Can you work these out from the model? Positions are in its coordinate system, mm. A direction names the side the tool comes from. Coordinates: 2 decimals unless noted, no trailing zeros. Loops run counter-clockwise (first coordinate to the right, second up) from the corner with the lowest first, then second, coordinate; pieces in that order, holes last. Notation, with made-up numbers: (83, 19.5) -> (133, 19.5) arc R5 ccw to (133, 23.5) -> close; hole circle Ø11 at (28.25, 18). An arc over 180 degrees is marked (long way). Put each result on its own line as item: value. Start each with the question number.
Item 1: Please list where these lines run through material, in increasing order: L1, parallel to X at y = 0, z = 13.75 (3 decimals); L2, parallel to X at y = -10, z = 15 (3 decimals); L3, parallel to Y at x = 48, z = 1.25 (3 decimals). Write a range as from..to.
Item 2: If we section it at D-D on x = -11.5: Please give me the cut outline in (y, z) (3 decimals).
Item 3: We'd pull the mould along Y, two halves only. Please class faces 6 (the flat face through (2.85, -26.07, 9.39)), 7 (the flat face through (-55.245, 1, 9)), 8 (the flat face through (1, 41.275, 9)), 9 (the flat face through (9.8, -46.06, 9.39)): pulls with the +Y half, pulls with the -Y half, needs draft (parallel to the pull), parting line crosses it, or undercut.
Item 4: Will these pins go through, and if not, where does the flat tip stop? P1, Ø4, axis at x = 46, z = 11.5, coming from the -Y side (3 decimals); P2, Ø8, axis at y = 17.5, z = 12, coming from the +X side.
Item 5: If we section it at A-A on x = -44.5: Please give me the cut outline in (y, z) (3 decimals), plus the area to 3 significant figures.
Item 6: If we section it at B-B on y = 25: Please give me the cut outline in (x, z) (3 decimals), plus the area to 3 significant figures.
Item 7: For faces 1 (the flat face through (35, -41.275, 9)), 2 (the flat face through (-39, -41.275, 9)), 3 (the flat face through (11.83, -25.95, 9.39)), 4 (the flat face through (20, 3, 0)), 5 (the flat face through (20, 3, 19.05)), which set-ups out of +Z, -Z, +X, -X, +Y, -Y let a thin tool reach every point of the face, with its end or its side?
Item 8: If we section it at C-C on z = 10.5: Please give me the cut outline in (x, y) (3 decimals).
```python
from build123d import *

# Parameters (mm, degrees)
F1_DEPTH = 19.05


with BuildPart() as f1:
    # F0 (on Top) → F1 (new body)
    with BuildSketch(Plane.XY):
        with BuildLine():
            ThreePointArc((95.083343, 10.795), (80.32549, 32.78101), (55.245, 41.275))
            Line((55.245, 41.275), (-55.245, 41.275))
            Line((-55.245, 41.275), (-55.245, -41.275))
            Line((-55.245, -41.275), (-21.336, -41.275))
            Line((-21.336, -41.275), (-7.865616, -41.275))
            Line((-7.865616, -41.275), (-20.82424, -28.316376))
            ThreePointArc((-20.82424, -28.316376), (-23.518744, 28.236761), (-17.489888, -28.058625))
            Line((-17.489888, -28.058625), (-4.273513, -41.275))
            Line((-4.273513, -41.275), (5.155756, -50.704269))
            Line((5.155756, -50.704269), (14.585024, -41.275))
            Line((14.585024, -41.275), (55.245, -41.275))
            ThreePointArc((55.245, -41.275), (80.32549, -32.78101), (95.083343, -10.795))
            ThreePointArc((95.083343, -10.795), (96.52, 0), (95.083343, 10.795))
        make_face()
        Polygon((16.381076, -30.498693), (7.40082, -39.478949), (-1.579437, -30.498693), (7.40082, -21.518437), align=None, mode=Mode.SUBTRACT)
        with BuildLine():
            ThreePointArc((84.427378, -1.27), (26.035, 0), (84.427378, 1.27))
            ThreePointArc((84.427378, 1.27), (84.455, 0), (84.427378, -1.27))
        make_face(mode=Mode.SUBTRACT)
        Polygon((-7.865616, -41.275), (-21.336, -41.275), (-3.375488, -59.235512), (3.359704, -52.50032), align=None)
    extrude(amount=F1_DEPTH)


solid = f1.part
```
Solutions:
1. L1: -55.245..-49.657, 6.985..26.035, 84.455..96.52
1. L2: -55.245..-47.833, 5.161..27.8, 82.69..95.29
1. L3: -41.275..-28.297, 28.297..41.275
2. outline: (-51.111, 0) -> (-37.641, 0) -> (-37.641, 19.05) -> (-51.111, 19.05) -> close; (-34.049, 0) -> (-26.558, 0) -> (-26.558, 19.05) -> (-34.049, 19.05) -> close; (26.558, 0) -> (41.275, 0) -> (41.275, 19.05) -> (26.558, 19.05) -> close
3. face 6: undercut
3. face 7: needs draft
3. face 8: pulls with the +Y half
3. face 9: pulls with the -Y half
4. P1: y = -41.275
4. P2: x = 94.25
5. outline: (-41.275, 0) -> (-16.294, 0) -> (-16.294, 19.05) -> (-41.275, 19.05) -> close; (16.294, 0) -> (41.275, 0) -> (41.275, 19.05) -> (16.294, 19.05) -> close
5. area: 952 mm^2
6. outline: (-55.245, 0) -> (-34.643, 0) -> (-34.643, 19.05) -> (-55.245, 19.05) -> close; (-8.029, 0) -> (40.138, 0) -> (40.138, 19.05) -> (-8.029, 19.05) -> close; (70.352, 0) -> (88.087, 0) -> (88.087, 19.05) -> (70.352, 19.05) -> close
6. area: 1,650 mm^2
7. face 1: +Z, -Z, +X, -Y
7. face 2: +Z, -Z, -X, -Y
7. face 3: +Z, -Z
7. face 4: -Z, +X, -X, +Y, -Y
7. face 5: +Z, +X, -X, +Y, -Y
8. outline: (-55.245, -41.275) -> (-21.336, -41.275) -> (-3.375, -59.236) -> (3.36, -52.5) -> (-20.824, -28.316) arc R28.321 cw (long way) to (-17.49, -28.059) -> (5.156, -50.704) -> (14.585, -41.275) -> (55.245, -41.275) arc R41.275 ccw to (95.083, -10.795) arc R41.275 ccw to (95.083, 10.795) arc R41.275 ccw to (55.245, 41.275) -> (-55.245, 41.275) -> close; hole (-1.579, -30.499) -> (7.401, -39.479) -> (16.381, -30.499) -> (7.401, -21.518) -> close; hole (84.427, -1.27) arc R29.21 ccw to (84.427, 1.27) arc R29.21 ccw (long way) to start
